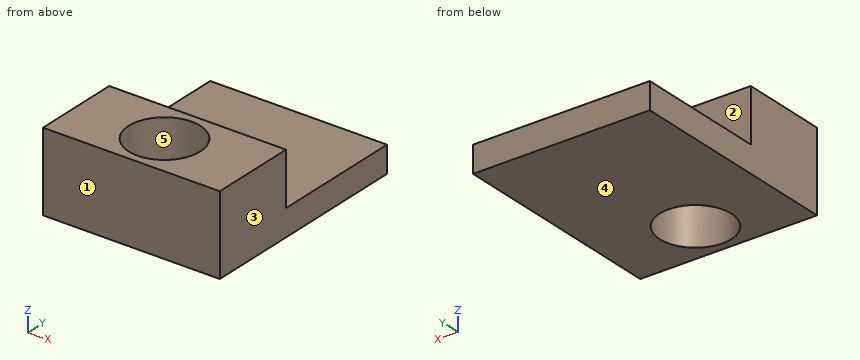
```python
from build123d import *

# Parameters (mm, degrees)
F0_W     = 20
F0_H     = 25
F1_DEPTH = 3
F3_DEPTH = 9
F4_R     = 4.05
F5_DEPTH = 9


with BuildPart() as f1:
    # F0 (on Top) → F1 (new body)
    with BuildSketch(Plane.XY):
        Rectangle(F0_W, F0_H)
    extrude(amount=F1_DEPTH)

    # F2 (on Top) → F3 (join)
    with BuildSketch(Plane.XY):
        Polygon((10, -2.6), (-10, -2.6), (-10, -6.8), (-10, -12.5), (10, -12.5), (10, -7.5), align=None)
    extrude(amount=F3_DEPTH)

    # F4 (on Top) → F5 (cut, through all)
    with BuildSketch(Plane.XY):
        with Locations((0, -7.55)):
            Circle(F4_R)
    extrude(amount=F5_DEPTH, mode=Mode.SUBTRACT)


solid = f1.part
```
For this review, take the finished solid that the model builds, in its own axes (mm). Face numbers are marked on the shaded views. A direction names the side the tool comes from. Coordinates: 2 decimals unless noted, no trailing zeros. Loops run counter-clockwise (first coordinate to the right, second up) from the corner with the lowest first, then second, coordinate; pieces in that order, holes last. Notation, with made-up numbers: (-3, -18.5) -> (35, -18.5) arc R24 ccw to (35, 3.5) -> close; hole circle Ø7 at (71, 7.25). An arc over 180 degrees is marked (long way). Return JSON: item names as keys, results as strings. Group by question number.
(1) Consider section A-A, the plane x = 0. Give the boundary of the cut face in (y, z).
(2) For pin 1 Ø2 at (x, z) = (2.5, 7.5) entering from +Y; pin 2 Ø8 at (x, y) = (2.5, -1) entering from +Z; pin 3 Ø7.5 at (x, y) = (4, 6.5) entering from +Z, all flat-tipped, find the tip position at first contact; note any pin that passes through.
(3) Mouldability with a two-part tool opening along X and no side actions: class the marked faces 3, 4 and 5 as pulls with the +X half, pulls with the -X half, needs draft (parallel to the pull), parting line crosses it, or undercut.
(4) To check wall thickness, follow L1, parallel to Y at x = 0, z = 3.25; L2, parallel to Y at x = 0, z = 2.25; L3, parallel to Z at x = 2.75, y = 5.5. State the ranges of each line that lie inside material, in increasing order.
(5) Consider section B-B, the plane y = -7.55. Give the boundary of the cut face in (x, z).
(6) Consider section D-D, the plane x = 5. Give the boundary of the cut face in (y, z), plus the area to 3 significant figures.
(7) Consider section C-C, the plane z = 3.5. Give the boundary of the cut face in (x, y).
(8) Tool access review of the marked faces 1 and 2: name each direction out of +Z, -Z, +X, -X, +Y, -Y from which nothing blocks a thin tool from reaching the whole face with its end or side.
Results below:
{
 "1": {"outline": "(-12.5, 0) -> (-11.6, 0) -> (-11.6, 9) -> (-12.5, 9) -> close; (-3.5, 0) -> (12.5, 0) -> (12.5, 3) -> (-2.6, 3) -> (-2.6, 9) -> (-3.5, 9) -> close"},
 "2": {"pin 1": "stops at y = -2.6", "pin 2": "stops at z = 9", "pin 3": "stops at z = 3"},
 "3": {"face 3": "pulls with the +X half", "face 4": "needs draft", "face 5": "undercut"},
 "4": {"L1": "y = -12.5 to -11.6, -3.5 to -2.6", "L2": "y = -12.5 to -11.6, -3.5 to 12.5", "L3": "z = 0 to 3"},
 "5": {"outline": "(-10, 0) -> (-4.05, 0) -> (-4.05, 9) -> (-10, 9) -> close; (4.05, 0) -> (10, 0) -> (10, 9) -> (4.05, 9) -> close"},
 "6": {"outline": "(-12.5, 0) -> (12.5, 0) -> (12.5, 3) -> (-2.6, 3) -> (-2.6, 9) -> (-12.5, 9) -> close", "area": "134 mm2"},
 "7": {"outline": "(-10, -12.5) -> (10, -12.5) -> (10, -2.6) -> (-10, -2.6) -> close; hole circle Ø8.1 at (0, -7.55)"},
 "8": {"face 1": "+Z, -Z, +X, -X, -Y", "face 2": "+Z, +X, -X, +Y"}
}
